For this review, use the dimensioned drawing (mm, ordinates from the lowest corner) and the shaded views. A direction names the side the tool comes from. Coordinates: 2 decimals unless noted, no trailing zeros. Write each loop counter-clockwise with the first axis right and the second up, starting at its lowest first coordinate (ties: lowest second). Pieces come first, ordered by that corner, then holes. Notation, with made-up numbers: M 87.25,12 L 113.25,12 A11 cw 113.25,26 Z; hole C -2.75,-28.75 d7. An arc over 180 degrees is marked long. Return JSON: item names as keys, results as strings.
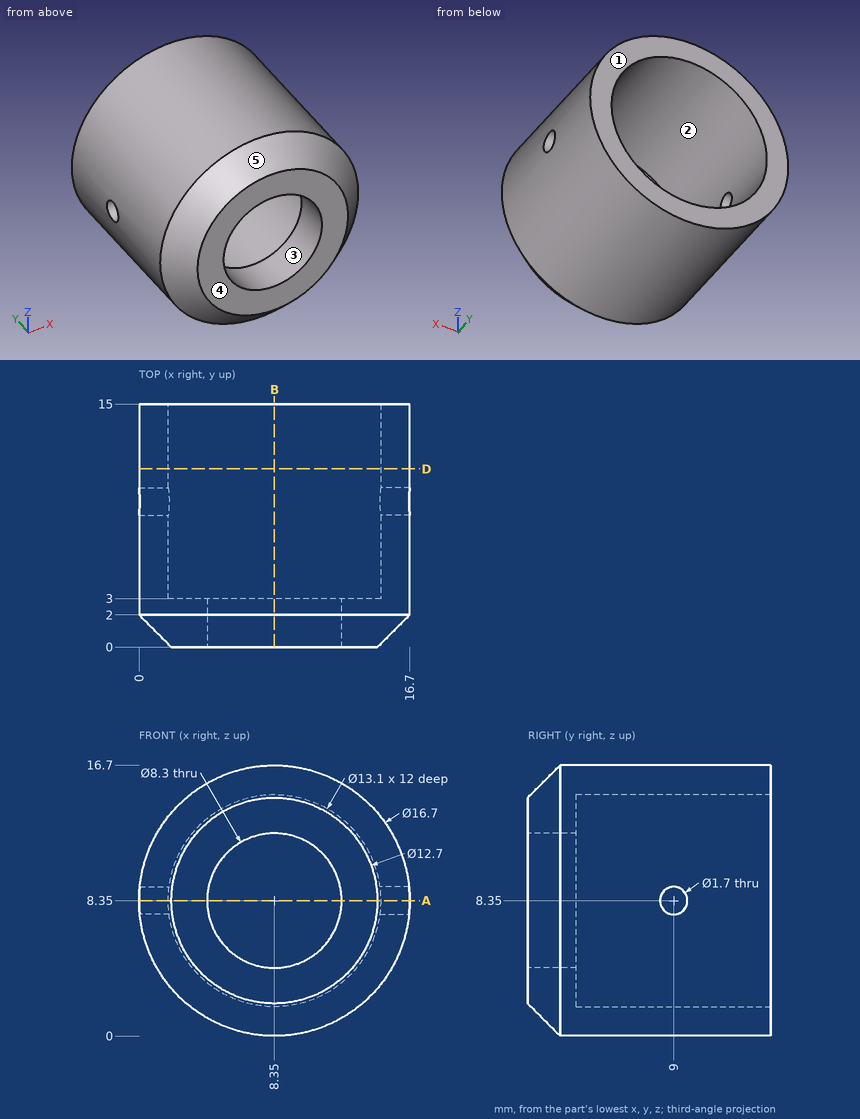
1. We need section D-D (y = 11). State the section outline as (x, z) points, plus the area to 3 significant figures.
Checks:
{"outline": "C 8.35,8.35 d16.7; hole C 8.35,8.35 d13.1", "area": "84.3 mm2"}
2. Clearance check with flat-ended pins moving along their axes: pin 1 Ø5 at (x, y) = (11.5, 13) entering from +Z; pin 2 Ø3 at (x, z) = (9, 12) entering from +Y; pin 3 Ø2 at (y, z) = (4, 10.5) entering from +X. State where each tip first meets the part, or that it passes through.
Checks:
{"pin 1": "z = 16.67", "pin 2": "y = 3", "pin 3": "x = 16.62"}
3. For the marked faces 1 and 2, list the 3-axis set-ups (+Z, -Z, +X, -X, +Y, -Y) from which the entire face can be reached by the end or side of a thin tool; tool diameter is ignored.
Checks:
{"face 1": "+Z, -Z, +X, -X, +Y", "face 2": "+Y"}
4. Wall thickness on L1, parallel to Z at x = 8.35, y = 8.5; L2, parallel to X at y = 6.75, z = 10.5: over which ranges is each line inside the solid? List them lowest first. Write a range as from..to.
Checks:
{"L1": "0..1.8, 14.9..16.7", "L2": "0.28..2.16, 14.54..16.42"}
5. We need section A-A (z = 8.35). State the section outline as (x, y) points, plus the area to 3 significant figures.
Checks:
{"outline": "M 0,2 L 2,0 L 4.2,0 L 4.2,3 L 1.8,3 L 1.8,8.15 L 0,8.15 Z; M 0,9.85 L 1.8,9.85 L 1.8,15 L 0,15 Z; M 12.5,0 L 14.7,0 L 16.7,2 L 16.7,8.15 L 14.9,8.15 L 14.9,3 L 12.5,3 Z; M 14.9,9.85 L 16.7,9.85 L 16.7,15 L 14.9,15 Z", "area": "58.3 mm2"}
6. Draft analysis for pull direction Z (two halves, no side actions). For the marked faces 3, 4 and 5, state which applies: +Z half, -Z half, draft (parallel to the pull), parting line (faces both ways), or undercut.
Checks:
{"face 3": "undercut", "face 4": "draft", "face 5": "parting line"}
7. We need section B-B (x = 8.35). State the section outline as (y, z) points.
Checks:
{"outline": "M 0,2 L 2,0 L 15,0 L 15,1.8 L 3,1.8 L 3,4.2 L 0,4.2 Z; M 0,12.5 L 3,12.5 L 3,14.9 L 15,14.9 L 15,16.7 L 2,16.7 L 0,14.7 Z"}
